Verification items for the finished model (mm, model axes). Coordinates: 2 decimals unless noted, no trailing zeros. Loops run counter-clockwise (first coordinate to the right, second up) from the corner with the lowest first, then second, coordinate; pieces in that order, holes last. Notation, with made-up numbers: (54, -37.5) - (78, -37.5) arc R21 ccw to (78, -19.5) - close; hole circle Ø11 at (31, 2.5). An arc over 180 degrees is marked (long way). One line per item, written item: value. Start each with the question number.
(1) Section check D-D (y = 65). Record the boundary of the cut face in (x, z), plus the area to 3 significant figures.
(2) Section check C-C (y = -41). Record the boundary of the cut face in (x, z) (3 decimals).
(3) Gauge pin test, flat ends, axial feed: P1, Ø1.5, axis at y = 32.5, z = 2, coming from the +X side; P2, Ø8, axis at x = -27.5, y = 77, coming from the +Z side; P3, Ø0.7, axis at x = 85, y = -69.5, coming from the +Z side; P4, Ø2, axis at y = -85, z = 8.5, coming from the +X side. Record the tip position at first contact, or that the pin passes through.
(4) Section check B-B (y = -80). Record the boundary of the cut face in (x, z) (3 decimals), plus the area to 3 significant figures.
(5) Thickness scan on probe 1 along Y at (x, z) = (9, 1.5) (3 decimals); probe 2 along Y at (x, z) = (65, 4); probe 3 along Y at (x, z) = (36, 4.5). Record the ranges inside material, lowest first. Write a range as [from, to].
(6) Section check A-A (x = -41). Record the boundary of the cut face in (y, z), plus the area to 3 significant figures.
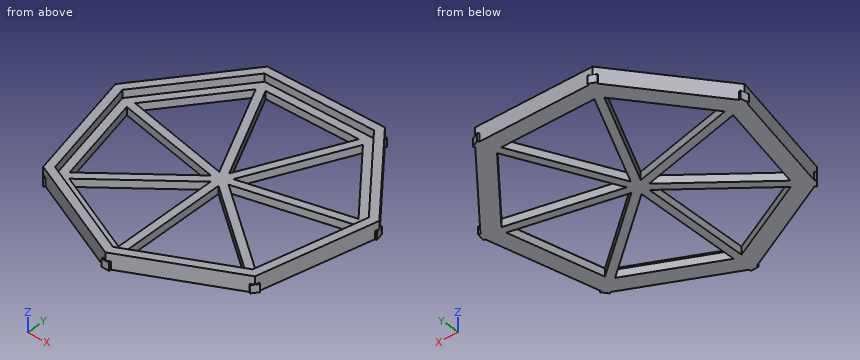
```python
from build123d import *

# Parameters (mm, degrees)
F1_E8_W   = 109.7644269796
F1_E8_H   = 6.35
F2_DEPTH  = 3.175
F1_E7_W   = 109.7644269796
F1_E7_H   = 6.35
F3_DEPTH  = 3.175
F4_E6_W   = 109.7644269796
F4_E6_H   = 6.35
F5_DEPTH  = 3.175
F4_E5_W   = 109.7644269796
F4_E5_H   = 6.35
F6_DEPTH  = 3.175
F7_E4_W   = 109.7644269796
F7_E4_H   = 6.35
F8_DEPTH  = 3.175
F7_E3_W   = 109.7644269796
F7_E3_H   = 6.35
F9_DEPTH  = 3.175
F10_E9_W  = 109.7644269796
F10_E9_H  = 6.35
F11_DEPTH = 3.175
F12_DEPTH = 12.7
F13_DEPTH = 6.35


with BuildPart() as f2:
    # F1_E8 (on explicit) → F2 (new body, symmetric)
    with BuildSketch(Plane(origin=(0, -109.7644269796, 0), x_dir=(0, 1, 0), z_dir=(1, 0, 0))):
        with Locations((54.8822134898, 3.175)):
            Rectangle(F1_E8_W, F1_E8_H)
    extrude(amount=F2_DEPTH, both=True)

    # F1_E7 (on explicit) → F3 (join, symmetric)
    with BuildSketch(Plane(origin=(85.8172846677, -68.4370008286, 0), x_dir=(-0.7818314825, 0.6234898019, 0), z_dir=(0.6234898019, 0.7818314825, 0))):
        with Locations((54.8822134898, 3.175)):
            Rectangle(F1_E7_W, F1_E7_H)
    extrude(amount=F3_DEPTH, both=True)

    # F4_E6 (on explicit) → F5 (join, symmetric)
    with BuildSketch(Plane(origin=(107.012403627, 24.4248828067, 0), x_dir=(-0.9749279122, -0.222520934, 0), z_dir=(-0.222520934, 0.9749279122, 0))):
        with Locations((54.8822134898, 3.175)):
            Rectangle(F4_E6_W, F4_E6_H)
    extrude(amount=F5_DEPTH, both=True)

    # F4_E5 (on explicit) → F6 (join, symmetric)
    with BuildSketch(Plane(origin=(47.625, 98.8943315118, 0), x_dir=(-0.4338837391, -0.9009688679, 0), z_dir=(-0.9009688679, 0.4338837391, 0))):
        with Locations((54.8822134898, 3.175)):
            Rectangle(F4_E5_W, F4_E5_H)
    extrude(amount=F6_DEPTH, both=True)

    # F7_E4 (on explicit) → F8 (join, symmetric)
    with BuildSketch(Plane(origin=(-47.625, 98.8943315118, 0), x_dir=(0.4338837391, -0.9009688679, 0), z_dir=(-0.9009688679, -0.4338837391, 0))):
        with Locations((54.8822134898, 3.175)):
            Rectangle(F7_E4_W, F7_E4_H)
    extrude(amount=F8_DEPTH, both=True)

    # F7_E3 (on explicit) → F9 (join, symmetric)
    with BuildSketch(Plane(origin=(-107.012403627, 24.4248828067, 0), x_dir=(0.9749279122, -0.222520934, 0), z_dir=(-0.222520934, -0.9749279122, 0))):
        with Locations((54.8822134898, 3.175)):
            Rectangle(F7_E3_W, F7_E3_H)
    extrude(amount=F9_DEPTH, both=True)

    # F10_E9 (on explicit) → F11 (join, symmetric)
    with BuildSketch(Plane(origin=(-85.8172846677, -68.4370008286, 0), x_dir=(0.7818314825, 0.6234898019, 0), z_dir=(0.6234898019, -0.7818314825, 0))):
        with Locations((54.8822134898, 3.175)):
            Rectangle(F10_E9_W, F10_E9_H)
    extrude(amount=F11_DEPTH, both=True)

    # F0 (on Top) → F12 (join)
    with BuildSketch(Plane.XY):
        Polygon((44.45, 92.3013760776), (47.625, 98.8943315118), (-47.625, 98.8943315118), (-44.45, 92.3013760776), align=None)
        Polygon((99.8782433852, 22.7965572862), (107.012403627, 24.4248828067), (47.625, 98.8943315118), (44.45, 92.3013760776), align=None)
        Polygon((80.0961323565, -63.8745341067), (85.8172846677, -68.4370008286), (107.012403627, 24.4248828067), (99.8782433852, 22.7965572862), align=None)
        Polygon((0, -109.7644269796), (85.8172846677, -68.4370008286), (80.0961323565, -63.8745341067), (0, -102.4467985143), align=None)
        Polygon((-85.8172846677, -68.4370008286), (0, -109.7644269796), (0, -102.4467985143), (-80.0961323565, -63.8745341067), align=None)
        Polygon((-107.012403627, 24.4248828067), (-85.8172846677, -68.4370008286), (-80.0961323565, -63.8745341067), (-99.8782433852, 22.7965572862), align=None)
        Polygon((-47.625, 98.8943315118), (-107.012403627, 24.4248828067), (-99.8782433852, 22.7965572862), (-44.45, 92.3013760776), align=None)
    extrude(amount=F12_DEPTH)

    # F0 (on Top) → F13 (join)
    with BuildSketch(Plane.XY):
        Polygon((92.7440831434, 21.1682317658), (99.8782433852, 22.7965572862), (44.45, 92.3013760776), (41.275, 85.7084206435), align=None)
        Polygon((41.275, 85.7084206435), (44.45, 92.3013760776), (-44.45, 92.3013760776), (-41.275, 85.7084206435), align=None)
        Polygon((-44.45, 92.3013760776), (-99.8782433852, 22.7965572862), (-92.7440831434, 21.1682317658), (-41.275, 85.7084206435), align=None)
        Polygon((-99.8782433852, 22.7965572862), (-80.0961323565, -63.8745341067), (-74.3749800453, -59.3120673848), (-92.7440831434, 21.1682317658), align=None)
        Polygon((-80.0961323565, -63.8745341067), (0, -102.4467985143), (0, -95.129170049), (-74.3749800453, -59.3120673848), align=None)
        Polygon((0, -102.4467985143), (80.0961323565, -63.8745341067), (74.3749800453, -59.3120673848), (0, -95.129170049), align=None)
        Polygon((74.3749800453, -59.3120673848), (80.0961323565, -63.8745341067), (99.8782433852, 22.7965572862), (92.7440831434, 21.1682317658), align=None)
    extrude(amount=F13_DEPTH)


solid = f2.part
```
Responses:
1. outline: (-74.65, 0) - (-57.79, 0) - (-57.79, 6.35) - (-66.22, 6.35) - (-66.22, 12.7) - (-74.65, 12.7) - close; (-34.83, 0) - (-27.78, 0) - (-27.78, 6.35) - (-34.83, 6.35) - close; (27.78, 0) - (34.83, 0) - (34.83, 6.35) - (27.78, 6.35) - close; (57.79, 0) - (74.65, 0) - (74.65, 12.7) - (66.22, 12.7) - (66.22, 6.35) - (57.79, 6.35) - close
1. area: 411 mm²
2. outline: (-92.08, 0) - (-78.555, 0) - (-78.555, 6.35) - (-85.317, 6.35) - (-85.317, 12.7) - (-92.08, 12.7) - close; (-56.505, 0) - (-46.32, 0) - (-46.32, 6.35) - (-56.505, 6.35) - close; (-3.175, 0) - (3.175, 0) - (3.175, 6.35) - (-3.175, 6.35) - close; (46.32, 0) - (56.505, 0) - (56.505, 6.35) - (46.32, 6.35) - close; (78.555, 0) - (92.08, 0) - (92.08, 12.7) - (85.317, 12.7) - (85.317, 6.35) - (78.555, 6.35) - close
3. P1: stops at x = 101.17
3. P2: passes through
3. P3: stops at z = 6.35
3. P4: stops at x = 53.5
4. outline: (-61.806, 0) - (-31.416, 0) - (-31.416, 6.35) - (-46.611, 6.35) - (-46.611, 12.7) - (-61.806, 12.7) - close; (-3.175, 0) - (3.175, 0) - (3.175, 6.35) - (-3.175, 6.35) - close; (31.416, 0) - (61.806, 0) - (61.806, 12.7) - (46.611, 12.7) - (46.611, 6.35) - (31.416, 6.35) - close
4. area: 619 mm²
5. probe 1: y = [-105.43, -90.795], [-11.238, -3.116], [-1.202, 5.311], [11.371, 26.006], [85.708, 98.894]
5. probe 2: y = [-78.46, -63.83], [-55.9, -47.77], [11.58, 18.09], [55.96, 77.11]
5. probe 3: y = [-92.43, -77.79], [-32.77, -24.65], [4.96, 11.47], [67.44, 82.07], [85.71, 98.89]
6. outline: (-90.02, 0) - (-75.38, 0) - (-75.38, 6.35) - (-82.7, 6.35) - (-82.7, 12.7) - (-90.02, 12.7) - close; (-36.76, 0) - (-28.64, 0) - (-28.64, 6.35) - (-36.76, 6.35) - close; (6.1, 0) - (12.61, 0) - (12.61, 6.35) - (6.1, 6.35) - close; (77.82, 0) - (98.89, 0) - (98.89, 12.7) - (92.3, 12.7) - (92.3, 6.35) - (77.82, 6.35) - close
6. area: 408 mm²
